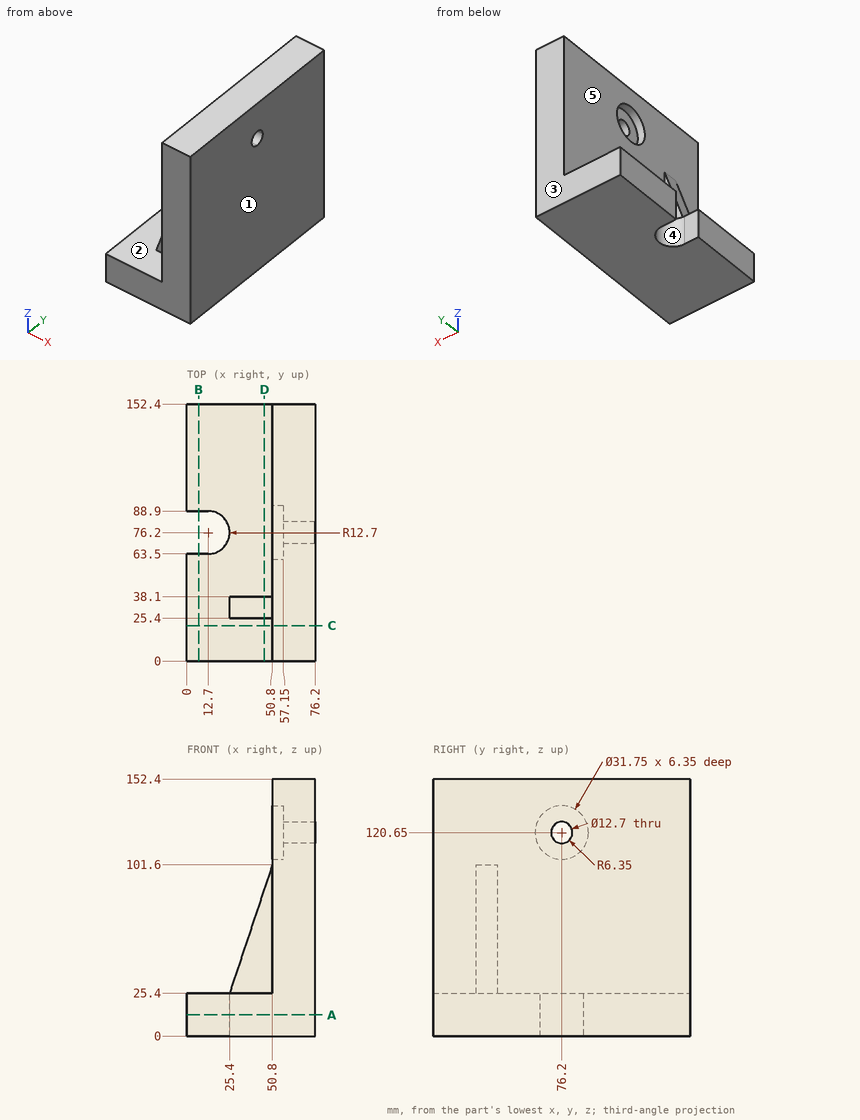
Geometry: see drawing. Coordinates: mm, zero at the bounding-box minimum. A direction names the side the tool comes from. Coordinates: 2 decimals unless noted, no trailing zeros. Loops run counter-clockwise (first coordinate to the right, second up) from the corner with the lowest first, then second, coordinate; pieces in that order, holes last. Notation, with made-up numbers: (33.5, 41) -> (73.5, 41) arc R23 ccw to (73.5, 64) -> close; hole circle Ø7 at (-20.75, 3.5). An arc over 180 degrees is marked (long way). Use a Markdown table: item, result.
1) Cut plane A-A (z = 12.5). Return the cut outline in (x, y).
Results found:
| item | result |
|---|---|
| outline | (0, 0) -> (76.2, 0) -> (76.2, 152.4) -> (0, 152.4) -> (0, 88.9) -> (12.7, 88.9) arc R12.7 cw to (12.7, 63.5) -> (0, 63.5) -> close |
2) Cut plane C-C (y = 21). Return the cut outline in (x, z).
Results found:
| item | result |
|---|---|
| outline | (0, 0) -> (76.2, 0) -> (76.2, 152.4) -> (50.8, 152.4) -> (50.8, 25.4) -> (0, 25.4) -> close |
3) Cut plane D-D (x = 46). Return the cut outline in (y, z).
Results found:
| item | result |
|---|---|
| outline | (0, 0) -> (152.4, 0) -> (152.4, 25.4) -> (38.1, 25.4) -> (38.1, 87.2) -> (25.4, 87.2) -> (25.4, 25.4) -> (0, 25.4) -> close |
4) Material intervals for line 1 along Y through (x, z) = (68, 120.65); line 2 along Z through (x, y) = (69, 76.2); line 3 along Z through (x, y) = (53.5, 76.2) (3 decimals), sorted ascending. Write a range as from..to.
Results found:
| item | result |
|---|---|
| line 1 | y = 0..69.85, 82.55..152.4 |
| line 2 | z = 0..114.3, 127..152.4 |
| line 3 | z = 0..104.775, 136.525..152.4 |
5) Cut plane B-B (x = 7). Return the cut outline in (y, z), then the cut area to 3 significant figures.
Results found:
| item | result |
|---|---|
| outline | (0, 0) -> (63.5, 0) -> (63.5, 25.4) -> (0, 25.4) -> close; (88.9, 0) -> (152.4, 0) -> (152.4, 25.4) -> (88.9, 25.4) -> close |
| area | 3,230 mm2 |
6) Contact query for flat-ended pins moving along their axis: pin 1 (12.5 mm diameter, centred on x = 41, z = 67.5, fed in from +Y); pin 2 (20.5 mm diameter, centred on x = 32, z = 59.5, fed in from -Y); pin 3 (5 mm diameter, centred on y = 104, z = 79.5, fed in from -X). Output: stop coordinate, or through.
Results found:
| item | result |
|---|---|
| pin 1 | stops at y = 38.1 |
| pin 2 | stops at y = 25.4 |
| pin 3 | stops at x = 50.8 |
7) Pull-direction query (Y, two-part tool) for the marked faces 3, 4 and 5; classes: released by +Y, released by -Y, zero draft, split by the parting line, or undercut.
Results found:
| item | result |
|---|---|
| face 3 | released by +Y |
| face 4 | undercut |
| face 5 | zero draft |
8) Access query for the marked faces 1 and 2. Directions: +Z, -Z, +X, -X, +Y, -Y. A direction counts if a zero-diameter tool reaches every point of the face in a straight line with its end or side. Return the directions, or none.
Results found:
| item | result |
|---|---|
| face 1 | +Z, -Z, +X, +Y, -Y |
| face 2 | +Z, -X |
